from build123d import *

# Parameters (mm, degrees)
SKETCH1_W             = 24.13
SKETCH1_H             = 22.352
BOSS_EXTRUDE1_DEPTH   = 3.81
SKETCH1_W_2           = 22.352
SKETCH1_H_2           = 24.13
BOSS_EXTRUDE1_2_DEPTH = 3.81
SKETCH2_W             = 22.352
SKETCH2_H             = 3.81
SKETCH2_W_2           = 3.81
SKETCH2_H_2           = 22.352
BOSS_EXTRUDE2_DEPTH   = 24.13
BOSS_EXTRUDE3_DEPTH   = 24.13
FILLET1_R             = 3.81


with BuildPart() as part:
    # Sketch1 → Boss-Extrude1 (new body)
    with BuildSketch(Plane(origin=(0, 0, 0), x_dir=(1, 0, 0), z_dir=(0, 1, 0))):
        with Locations((37.973, -38.862)):
            Rectangle(SKETCH1_W, SKETCH1_H)
    extrude(amount=BOSS_EXTRUDE1_DEPTH)



with BuildPart() as body_2:
    # Sketch1 → Boss-Extrude1 2 (new body)
    with BuildSketch(Plane(origin=(0, 0, 0), x_dir=(1, 0, 0), z_dir=(0, 1, 0))):
        with Locations((11.176, -12.065)):
            Rectangle(SKETCH1_W_2, SKETCH1_H_2)
    extrude(amount=BOSS_EXTRUDE1_2_DEPTH)


with BuildPart() as part_1:
    add(part.part)

    add(body_2.part)  # Boss-Extrude2 merges body 2
    # Sketch2 → Boss-Extrude2 (add)
    with BuildSketch(Plane(origin=(0, 3.81, 0), x_dir=(1, 0, 0), z_dir=(0, 1, 0))):
        with Locations((11.176, -1.905)):
            Rectangle(SKETCH2_W, SKETCH2_H)
        with Locations((48.133, -38.862)):
            Rectangle(SKETCH2_W_2, SKETCH2_H_2)
    extrude(amount=BOSS_EXTRUDE2_DEPTH)

    # Sketch3 → Boss-Extrude3 (add)
    with BuildSketch(Plane.XZ):
        Polygon((22.352, 27.686), (50.038, 27.686), (50.038, 31.496), (18.542, 31.496), (18.542, 0), (22.352, 0), align=None)
    extrude(amount=BOSS_EXTRUDE3_DEPTH)

    # Fillet1
    fillet1_edges = [part_1.edges().sort_by_distance(p)[0] for p in [
        (18.542, -12.065, 31.496),
    ]]
    fillet(fillet1_edges, radius=FILLET1_R)


solid = part_1.part
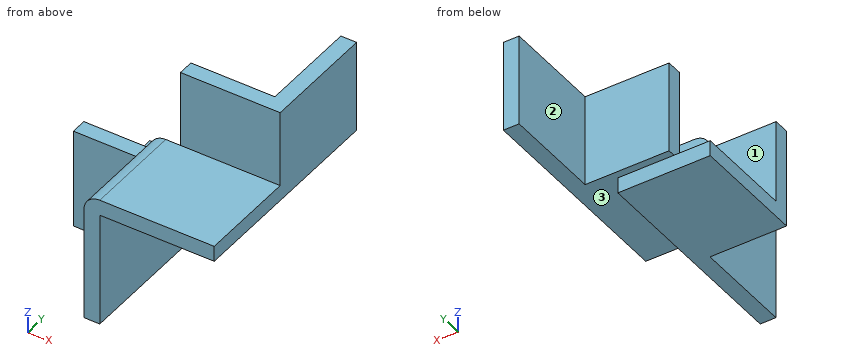
The model under review builds one solid part; all positions refer to its coordinate system, in mm. Face numbers are marked on the shaded views. A direction names the side the tool comes from. Coordinates: 2 decimals unless noted, no trailing zeros. Write each loop counter-clockwise with the first axis right and the second up, starting at its lowest first coordinate (ties: lowest second). Pieces come first, ordered by that corner, then holes. Notation, with made-up numbers: (20.25, -23.5) - (27.25, -23.5) arc R23 cw to (27.25, -3.5) - close; hole circle Ø7 at (48, 6). An arc over 180 degrees is marked (long way). Answer as a JSON object with one key per item and string values. Group by question number.
1. To check wall thickness, follow probe 1 along Y at (x, z) = (39, 41.5); probe 2 along X at (y, z) = (-15, 15). State the ranges of each line that lie inside material, in increasing order.
2. Machinability: for the marked faces 1, 2 and 3, which of the approach directions +Z, -Z, +X, -X, +Y, -Y give a long, thin tool a straight path to every point of the face, cutting with its end or side? Answer none if there is none.
3. Add section A-A (y = 13). Give the boundary of the cut face in (x, z), plus the area to 3 significant figures.
4. Add section C-C (x = 13). Give the boundary of the cut face in (y, z).
5. Clearance check with flat-ended pins moving along their axes: pin 1 Ø11 at (x, y) = (7.5, 20.5) entering from +Z; pin 2 Ø24.5 at (y, z) = (14, 42.5) entering from -X; pin 3 Ø4 at (x, y) = (7, 1.5) entering from +Z; pin 4 Ø12 at (x, z) = (39, 17) entering from +Y. State where each tip first meets the part, or that it passes through.
6. Add section B-B (z = 32.5). Give the boundary of the cut face in (x, y).
7. Add section D-D (y = -11.5). Give the boundary of the cut face in (x, z), plus the area to 3 significant figures.
Findings:
{
 "1": {"probe 1": "0 to 3.81", "probe 2": "18.54 to 22.35"},
 "2": {"face 1": "+Z, +X, -X, +Y", "face 2": "+Z, -Z, -X, +Y", "face 3": "-Z, +X, +Y, -Y"},
 "3": {"outline": "(0, 0) - (22.35, 0) - (22.35, 3.81) - (0, 3.81) - close; (46.23, 27.69) - (50.04, 27.69) - (50.04, 50.04) - (46.23, 50.04) - close", "area": "170 mm²"},
 "4": {"outline": "(0, 0) - (27.94, 0) - (27.94, 3.81) - (3.81, 3.81) - (3.81, 24.13) - (0, 24.13) - close"},
 "5": {"pin 1": "z = 3.81", "pin 2": "x = 25.91", "pin 3": "z = 24.13", "pin 4": "through"},
 "6": {"outline": "(25.91, 0) - (50.04, 0) - (50.04, 27.94) - (46.23, 27.94) - (46.23, 3.81) - (25.91, 3.81) - close"},
 "7": {"outline": "(18.54, 0) - (22.35, 0) - (22.35, 27.69) - (50.04, 27.69) - (50.04, 31.5) - (22.35, 31.5) arc R3.81 ccw to (18.54, 27.69) - close", "area": "222 mm²"}
}
